The model under review builds one solid part; all positions refer to its coordinate system, in mm. A direction names the side the tool comes from. Give positions to 0.01 mm unless a question says otherwise; leave off trailing zeros. Write each loop counter-clockwise with the first axis right and the second up, starting at its lowest first coordinate (ties: lowest second). Pieces come first, ordered by that corner, then holes.
from build123d import *

# Parameters (mm, degrees)
BASE_R              = 1.55
BOSS_EXTRUDE1_DEPTH = 2.5
SKETCH1_3_W         = 4.5
SKETCH1_3_H         = 4.5
SKETCH1_3_R         = 1.625
BOSS_EXTRUDE2_DEPTH = 0.65
SKETCH1_4_W         = 4
SKETCH1_4_H         = 5.25
BOSS_EXTRUDE3_DEPTH = 0.25
FILLET1_R           = 2.5


with BuildPart() as part:
    # Base → Boss-Extrude1 (new body)
    with BuildSketch(Plane(origin=(0, 0, 0), x_dir=(1, 0, 0), z_dir=(0, 1, 0))):
        Polygon((-7.5, -7.5), (-2, -7.5), (-2, -2.25), (-2.25, -2.25), (-2.25, 2.25), (2.25, 2.25), (2.25, -2.25), (2, -2.25), (2, -7.5), (7.5, -7.5), (7.5, 7.5), (-7.5, 7.5), align=None)
        with Locations(Location((-4.75, -4.75, 0), (0, 0, 270))):
            Circle(BASE_R, mode=Mode.SUBTRACT)
        with Locations(Location((4.75, -4.75, 0), (0, 0, 270))):
            Circle(BASE_R, mode=Mode.SUBTRACT)
        with Locations(Location((-4.75, 4.75, 0), (0, 0, 270))):
            Circle(BASE_R, mode=Mode.SUBTRACT)
        with Locations(Location((4.75, 4.75, 0), (0, 0, 270))):
            Circle(BASE_R, mode=Mode.SUBTRACT)
    extrude(amount=BOSS_EXTRUDE1_DEPTH)

    # Sketch1_3 → Boss-Extrude2 (add)
    with BuildSketch(Plane(origin=(0, 0, 0), x_dir=(1, 0, 0), z_dir=(0, 1, 0))):
        Rectangle(SKETCH1_3_W, SKETCH1_3_H)
        with Locations(Location((0, 0, 0), (0, 0, 270))):
            Circle(SKETCH1_3_R, mode=Mode.SUBTRACT)
    extrude(amount=BOSS_EXTRUDE2_DEPTH)

    # Sketch1_4 → Boss-Extrude3 (add)
    with BuildSketch(Plane(origin=(0, 0, 0), x_dir=(1, 0, 0), z_dir=(0, 1, 0))):
        with Locations((0, -4.875)):
            Rectangle(SKETCH1_4_W, SKETCH1_4_H)
    extrude(amount=BOSS_EXTRUDE3_DEPTH)

    # Fillet1
    fillet1_edges = [part.edges().sort_by_distance(p)[0] for p in [
        (-7.5, 1.25, 7.5),
        (-7.5, 1.25, -7.5),
        (7.5, 1.25, -7.5),
        (7.5, 1.25, 7.5),
    ]]
    fillet(fillet1_edges, radius=FILLET1_R)


solid = part.part
1) Tool access review of faces 4 (the flat face through (-2.25, 2, 0)), 5 (the flat face through (0, 0.25, 5)), 6 (the flat face through (0, 1, -7.5)): name each direction out of +Z, -Z, +X, -X, +Y, -Y from which nothing blocks a thin tool from reaching the whole face with its end or side.
2) Consider section A-A, the plane y = 1.65. Give the boundary of the cut face in (x, z), then the cut area to 3 significant figures.
3) Consider section D-D, the plane x = 4.75. Give the boundary of the cut face in (y, z).
4) Consider section B-B, the plane z = 4.75. Give the boundary of the cut face in (x, y), then the cut area to 3 significant figures.
5) To check wall thickness, follow probe 1 along X at (y, z) = (0.75, 4.75); probe 2 along X at (y, z) = (1.55, -4.75); probe 3 along X at (y, z) = (1.75, -1). State the ranges of each line that lie inside material, in increasing order.
6) Insertion check: pin 1 (2 mm diameter, centred on x = -0.5, z = 5.5, fed in from +Y); pin 2 (1.5 mm diameter, centred on x = 6, y = 1, fed in from +Z). Each pin has a flat end and moves straight along its axis. Give the tip position at first contact, or say it passes through.
7) The part is to be moulded in two halves that separate along X. For faces 1 (the cylindrical face through (-6.748, 1.268, 6.787)), 2 (the flat face through (-2, 0.65, -1)), 3 (the flat face through (7.5, 1, 0)), say which applies: +X half, -X half, draft (parallel to the pull), parting line (faces both ways), or undercut.
8) Consider section C-C, the plane x = 0. Give the boundary of the cut face in (y, z) (3 decimals), then the cut area to 4 significant figures.
Answer block:
1. face 4: +Y
1. face 5: +Z, +Y
1. face 6: -Z, +X, -X, +Y, -Y
2. outline: (-7.5, -5) arc R2.5 ccw to (-5, -7.5) - (5, -7.5) arc R2.5 ccw to (7.5, -5) - (7.5, 5) arc R2.5 ccw to (5, 7.5) - (2, 7.5) - (2, 2.25) - (2.25, 2.25) - (2.25, -2.25) - (-2.25, -2.25) - (-2.25, 2.25) - (-2, 2.25) - (-2, 7.5) - (-5, 7.5) arc R2.5 ccw to (-7.5, 5) - close; hole circle Ø3.1 at (-4.75, -4.75); hole circle Ø3.1 at (-4.75, 4.75); hole circle Ø3.1 at (4.75, -4.75); hole circle Ø3.1 at (4.75, 4.75)
2. area: 148 mm2
3. outline: (0, -7.5) - (2.5, -7.5) - (2.5, -6.3) - (0, -6.3) - close; (0, -3.2) - (2.5, -3.2) - (2.5, 3.2) - (0, 3.2) - close; (0, 6.3) - (2.5, 6.3) - (2.5, 7.5) - (0, 7.5) - close
4. outline: (-7.5, 0) - (-6.3, 0) - (-6.3, 2.5) - (-7.5, 2.5) - close; (-3.2, 0) - (3.2, 0) - (3.2, 2.5) - (2, 2.5) - (2, 0.25) - (-2, 0.25) - (-2, 2.5) - (-3.2, 2.5) - close; (6.3, 0) - (7.5, 0) - (7.5, 2.5) - (6.3, 2.5) - close
4. area: 13.0 mm2
5. probe 1: x = -7.5 to -6.3, -3.2 to -2, 2 to 3.2, 6.3 to 7.5
5. probe 2: x = -7.5 to -6.3, -3.2 to 3.2, 6.3 to 7.5
5. probe 3: x = -7.5 to -2.25, 2.25 to 7.5
6. pin 1: stops at y = 0.25
6. pin 2: stops at z = 7.49
7. face 1: -X half
7. face 2: undercut
7. face 3: +X half
8. outline: (0, -7.5) - (2.5, -7.5) - (2.5, -2.25) - (0.65, -2.25) - (0.65, -1.625) - (0, -1.625) - close; (0, 1.625) - (0.65, 1.625) - (0.65, 2.25) - (0.25, 2.25) - (0.25, 7.5) - (0, 7.5) - close
8. area: 15.25 mm2
